```python
from build123d import *

# Parameters (mm, degrees)
F1_DEPTH = 44.45
F2_W     = 38.1
F2_H     = 38.1
F3_DEPTH = 538.957237


with BuildPart() as f1:
    # F0 (on Front) → F1 (new body)
    with BuildSketch(Plane.XZ):
        Polygon((0, 44.45), (0, 0), (538.956237, 0), (533.4, 44.45), align=None)
    extrude(amount=F1_DEPTH)

    # F2 (on face) → F3 (cut, through all)
    with BuildSketch(Plane(origin=(0, 0, 0), x_dir=(0, -1, 0), z_dir=(-1, 0, 0))):
        with Locations((22.225, 22.225)):
            Rectangle(F2_W, F2_H)
    extrude(amount=-F3_DEPTH, mode=Mode.SUBTRACT)


solid = f1.part
```
Input: part model. Units: mm. Frame: model coordinates. A direction names the side the tool comes from. Coordinates: 2 decimals unless noted, no trailing zeros. Write each loop counter-clockwise with the first axis right and the second up, starting at its lowest first coordinate (ties: lowest second). Pieces come first, ordered by that corner, then holes.
1) Section A-A on x = 311. Output: boundary loops of the cut face in (y, z) (3 decimals), and give its area (3 significant figures).
2) Section B-B on y = -23. Output: boundary loops of the cut face in (x, z) (3 decimals).
3) Mould query, pull axis Z, two halves, no side actions, for faces 3 (the flat face through (266, -41.275, 22)), 4 (the flat face through (266, -22, 0)), 5 (the flat face through (266, 0, 23)). Classes: pulls with the +Z half, pulls with the -Z half, needs draft (parallel to the pull), parting line crosses it, or undercut.
4) Material intervals for line 1 along Z through (x, y) = (468.5, -21.5) (3 decimals); line 2 along Y through (x, z) = (293.5, 11) (3 decimals), sorted ascending.
5) Section C-C on z = 17. Output: boundary loops of the cut face in (x, y) (3 decimals), and give its area (3 significant figures).
6) Set-up query: faces 1 (the flat face through (263, -22, 41.275)), 2 (the flat face through (0, -22, 3)). Return all of +Z, -Z, +X, -X, +Y, -Y with unobstructed straight access to the full face (end or side cutting, diameter ignored); none if empty.
Check result:
1. outline: (-44.45, 0) - (0, 0) - (0, 44.45) - (-44.45, 44.45) - close; hole (-41.275, 3.175) - (-3.175, 3.175) - (-3.175, 41.275) - (-41.275, 41.275) - close
1. area: 524 mm2
2. outline: (0, 0) - (538.956, 0) - (538.559, 3.175) - (0, 3.175) - close; (0, 41.275) - (533.797, 41.275) - (533.4, 44.45) - (0, 44.45) - close
3. face 3: undercut
3. face 4: pulls with the -Z half
3. face 5: needs draft
4. line 1: z = 0 to 3.175, 41.275 to 44.45
4. line 2: y = -44.45 to -41.275, -3.175 to 0
5. outline: (0, -44.45) - (536.831, -44.45) - (536.831, -41.275) - (0, -41.275) - close; (0, -3.175) - (536.831, -3.175) - (536.831, 0) - (0, 0) - close
5. area: 3,410 mm2
6. face 1: +X, -X
6. face 2: +Z, -Z, -X, +Y, -Y
